Could you check a few things on this model? Use its own coordinates, in mm. Face numbers are marked on the shaded views. Give positions to 0.01 mm unless a question says otherwise; leave off trailing zeros. Write each loop counter-clockwise with the first axis right and the second up, starting at its lowest first coordinate (ties: lowest second). Pieces come first, ordered by that corner, then holes. Notation, with made-up numbers: (16.5, -3.75) - (75.5, -3.75) arc R22 ccw to (75.5, 35.25) - close; hole circle Ø7 at (67.25, 35.5). An arc over 180 degrees is marked (long way). Answer in a Markdown table with one row per item.
from build123d import *

# Parameters (mm, degrees)
CROQUIS1_R              = 1
SALIENTE_EXTRUIR1_DEPTH = 0.2
CROQUIS2_R              = 1.25
CROQUIS2_R_2            = 1
SALIENTE_EXTRUIR2_DEPTH = 0.2


with BuildPart() as part:
    # Croquis1 → Saliente-Extruir1 (new body)
    with BuildSketch(Plane.XY):
        with BuildLine():
            Line((0.5, 1.414213562), (0.75, 3.5))
            Line((0.75, 3.5), (0.25, 6))
            Line((0.25, 6), (1.25, 8))
            Line((1.25, 8), (0.125, 10.5))
            Line((0.125, 10.5), (0.125, 14))
            Line((0.125, 14), (-0.125, 14))
            Line((-0.125, 14), (-0.125, 10.5))
            Line((-0.125, 10.5), (-1.25, 8))
            Line((-1.25, 8), (-0.25, 6))
            Line((-0.25, 6), (-0.75, 3.5))
            Line((-0.75, 3.5), (-0.5, 1.414213562))
            ThreePointArc((-0.5, 1.414213562), (0, -1.5), (0.5, 1.414213562))
        make_face()
        Circle(CROQUIS1_R, mode=Mode.SUBTRACT)
        Polygon((0, 6), (1, 8), (0, 10.5), (-1, 8), align=None, mode=Mode.SUBTRACT)
    extrude(amount=SALIENTE_EXTRUIR1_DEPTH)

    # Croquis2 → Saliente-Extruir2 (add)
    with BuildSketch(Plane(origin=(0, 0, 0), x_dir=(-1, 0, 0), z_dir=(0, 0, -1))):
        Circle(CROQUIS2_R)
        Circle(CROQUIS2_R_2, mode=Mode.SUBTRACT)
    extrude(amount=SALIENTE_EXTRUIR2_DEPTH)


solid = part.part
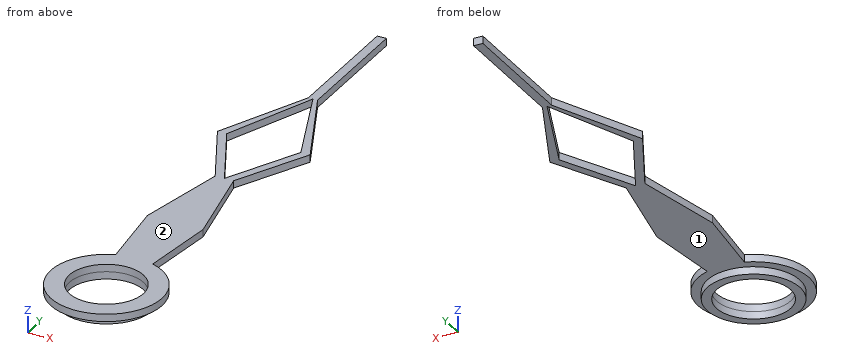
1) Imagine slicing it at A-A (z = 0.1). List the corners of the cut face in (x, y) for me (3 decimals).
Check values:
| item | result |
|---|---|
| outline | (-1.25, 8) - (-0.25, 6) - (-0.75, 3.5) - (-0.5, 1.414) arc R1.5 ccw (long way) to (0.5, 1.414) - (0.75, 3.5) - (0.25, 6) - (1.25, 8) - (0.125, 10.5) - (0.125, 14) - (-0.125, 14) - (-0.125, 10.5) - close; hole circle Ø2 at (0, 0); hole (-1, 8) - (0, 6) - (1, 8) - (0, 10.5) - close |
2) Imagine slicing it at D-D (y = 11.25). List the corners of the cut face in (x, z) for me (3 decimals), then the cut area to 3 significant figures.
Check values:
| item | result |
|---|---|
| outline | (-0.125, 0) - (0.125, 0) - (0.125, 0.2) - (-0.125, 0.2) - close |
| area | 0.0500 mm2 |
3) If I drill on line 1 (X direction, y = 0, z = 0.05); line 2 (Z direction, x = 0.3, y = 5); line 3 (Y direction, x = 0.25, z = -0.1), over which ranges is the centre line in solid material (lowest first)?
Check values:
| item | result |
|---|---|
| line 1 | x = -1.5 to -1, 1 to 1.5 |
| line 2 | z = 0 to 0.2 |
| line 3 | y = -1.22 to -0.97, 0.97 to 1.22 |
4) Imagine slicing it at C-C (y = 0). List the corners of the cut face in (x, z) for me, then the cut area to 3 significant figures.
Check values:
| item | result |
|---|---|
| outline | (-1.5, 0) - (-1.25, 0) - (-1.25, -0.2) - (-1, -0.2) - (-1, 0.2) - (-1.5, 0.2) - close; (1, -0.2) - (1.25, -0.2) - (1.25, 0) - (1.5, 0) - (1.5, 0.2) - (1, 0.2) - close |
| area | 0.300 mm2 |
5) Will these pins go through, and if not, where does the flat tip stop? P1, Ø1.5, axis at x = -1, y = 6, coming from the -Z side; P2, Ø1.6, axis at x = 0, y = 0, coming from the -Z side.
Check values:
| item | result |
|---|---|
| P1 | stops at z = 0 |
| P2 | passes through |
6) We'd pull the mould along Z, two halves only. Please class the marked faces 1 and 2: +Z half, -Z half, draft (parallel to the pull), parting line (faces both ways), or undercut.
Check values:
| item | result |
|---|---|
| face 1 | -Z half |
| face 2 | +Z half |
7) Imagine slicing it at B-B (y = 7.25). List the corners of the cut face in (x, z) for me (3 decimals).
Check values:
| item | result |
|---|---|
| outline | (-0.875, 0) - (-0.625, 0) - (-0.625, 0.2) - (-0.875, 0.2) - close; (0.625, 0) - (0.875, 0) - (0.875, 0.2) - (0.625, 0.2) - close |
